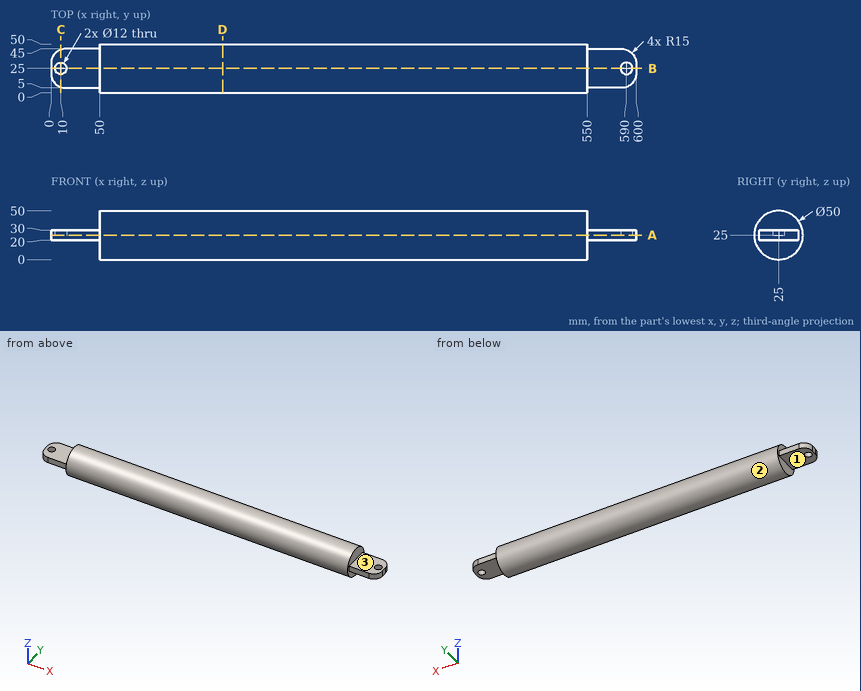
Design review of the part shown in the three views and the two pictorial views. Dimensions are in mm from the part's minimum x, y and z. A direction names the side the tool comes from. Coordinates: 2 decimals unless noted, no trailing zeros. Write each loop counter-clockwise with the first axis right and the second up, starting at its lowest first coordinate (ties: lowest second). Pieces come first, ordered by that corner, then holes.
1) We need section B-B on y = 25. State the section outline as (x, z) points, then the cut area to 3 significant figures.
2) We need section D-D on x = 176. State the section outline as (y, z) points, then the cut area to 3 significant figures.
3) Machinability: for the marked faces 1, 2 and 3, which of the approach directions +Z, -Z, +X, -X, +Y, -Y give a long, thin tool a straight path to every point of the face, cutting with its end or side? Answer none if there is none.
4) We need section C-C on x = 10. State the section outline as (y, z) points, then the cut area to 3 significant figures.
5) To check wall thickness, follow probe 1 along X at (y, z) = (4.5, 23); probe 2 along Y at (x, z) = (10, 26.5); probe 3 along Z at (x, y) = (25.5, 10.5). State the ranges of each line that lie inside material, in increasing order.
6) We need section A-A on z = 25. State the section outline as (x, y) points.
7) Clearance check with flat-ended pins moving along their axes: pin 1 Ø5 at (x, z) = (576, 27.5) entering from +Y; pin 2 Ø1 at (x, z) = (185, 12.5) entering from +Y; pin 3 Ø7 at (x, y) = (590, 25) entering from +Z; pin 4 Ø8 at (y, z) = (38, 25.5) entering from +X. State where each tip first meets the part, or that it passes through.
Answer list:
1. outline: (0, 20) - (4, 20) - (4, 30) - (0, 30) - close; (16, 20) - (50, 20) - (50, 0) - (550, 0) - (550, 20) - (584, 20) - (584, 30) - (550, 30) - (550, 50) - (50, 50) - (50, 30) - (16, 30) - close; (596, 20) - (600, 20) - (600, 30) - (596, 30) - close
1. area: 25,800 mm2
2. outline: circle Ø50 at (25, 25)
2. area: 1,960 mm2
3. face 1: -Z, -X, +Y, -Y
3. face 2: +X, -X
3. face 3: +Z, +X, +Y, -Y
4. outline: (5.86, 20) - (19, 20) - (19, 30) - (5.86, 30) - close; (31, 20) - (44.14, 20) - (44.14, 30) - (31, 30) - close
4. area: 263 mm2
5. probe 1: x = 50 to 550
5. probe 2: y = 5.86 to 19, 31 to 44.14
5. probe 3: z = 20 to 30
6. outline: (0, 20) arc R15 ccw to (15, 5) - (50, 5) - (50, 0) - (550, 0) - (550, 5) - (585, 5) arc R15 ccw to (600, 20) - (600, 30) arc R15 ccw to (585, 45) - (550, 45) - (550, 50) - (50, 50) - (50, 45) - (15, 45) arc R15 ccw to (0, 30) - close; hole circle Ø12 at (10, 25); hole circle Ø12 at (590, 25)
7. pin 1: stops at y = 45
7. pin 2: stops at y = 46.93
7. pin 3: passes through
7. pin 4: stops at x = 599.46
